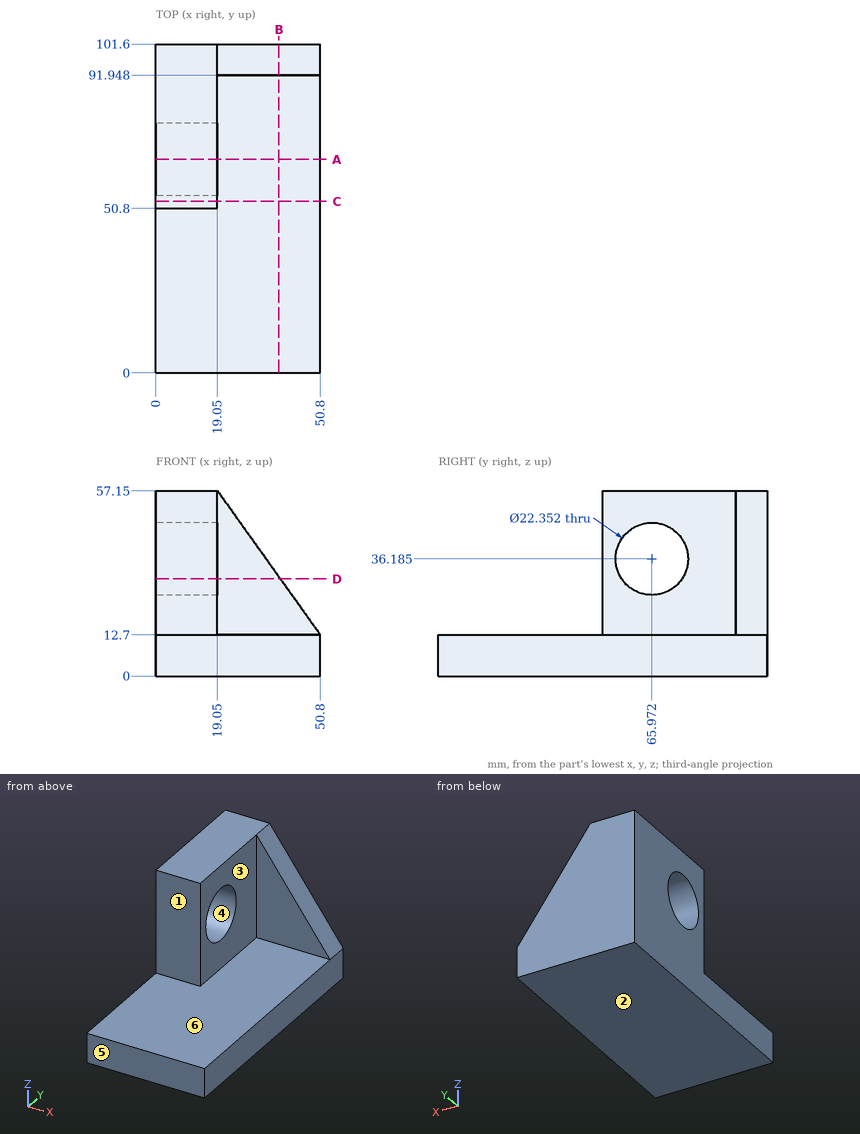
Verification items for this drawing (mm, ordinates from the low corner). A direction names the side the tool comes from. Give positions to 0.01 mm unless a question says otherwise; leave off trailing zeros. Loops run counter-clockwise (first coordinate to the right, second up) from the corner with the lowest first, then second, coordinate; pieces in that order, holes last. Notation, with made-up numbers: M 31.25,-33 L 49.25,-33 A27 cw 49.25,-16 Z; hole C 62.25,51.25 d8. An arc over 180 degrees is marked long. Answer as a JSON object with one key per item and string values. Group by question number.
Q1. Release check for a two-part mould opening along Y. For the marked faces 4, 5 and 6 record: released by +Y, released by -Y, zero draft, split by the parting line, or undercut.
Q2. Cross-section at B-B on x = 38. Record the cut outline in (y, z), then the cut area to 3 significant figures.
Q3. Access from +Z, -Z, +X, -X, +Y, -Y to the whole of each face (thin tool, end or side, straight path). Record for the marked faces 1, 2 and 3.
Q4. Cross-section at A-A on y = 66. Record the cut outline in (x, z).
Q5. Cross-section at C-C on y = 53. Record the cut outline in (x, z), then the cut area to 3 significant figures.
Q6. Go/stop test with flat-tipped pins: P1, Ø3, axis at x = 20.5, z = 42.5, coming from the -Y side; P2, Ø1.5, axis at y = 73.5, z = 16, coming from the +X side; P3, Ø1, axis at x = 24.5, y = 38.5, coming from the +Z side. Record where each tip stops, or that it passes through.
Q7. Cross-section at D-D on z = 30. Record the cut outline in (x, y).
Q8. Material ranges on line 1 along Y through (x, z) = (28, 37); line 2 along X through (y, z) = (83.5, 32.5); line 3 along Z through (x, y) = (14, 44), recorded low to high. Write a range as [from, to].
Evaluation:
{
 "1": {"face 4": "undercut", "face 5": "released by -Y", "face 6": "zero draft"},
 "2": {"outline": "M 0,0 L 101.6,0 L 101.6,30.62 L 91.95,30.62 L 91.95,12.7 L 0,12.7 Z", "area": "1,460 mm2"},
 "3": {"face 1": "+Z, +X, -X, -Y", "face 2": "-Z, +X, -X, +Y, -Y", "face 3": "+Z, +X, -Y"},
 "4": {"outline": "M 0,0 L 50.8,0 L 50.8,12.7 L 19.05,12.7 L 19.05,25.01 L 0,25.01 Z; M 0,47.36 L 19.05,47.36 L 19.05,57.15 L 0,57.15 Z"},
 "5": {"outline": "M 0,0 L 50.8,0 L 50.8,12.7 L 19.05,12.7 L 19.05,57.15 L 0,57.15 Z", "area": "1,490 mm2"},
 "6": {"P1": "stops at y = 50.8", "P2": "stops at x = 19.05", "P3": "stops at z = 12.7"},
 "7": {"outline": "M 0,50.8 L 19.05,50.8 L 19.05,56.66 L 0,56.66 Z; M 0,75.28 L 19.05,75.28 L 19.05,91.95 L 38.44,91.95 L 38.44,101.6 L 0,101.6 Z"},
 "8": {"line 1": "y = [91.95, 101.6]", "line 2": "x = [0, 19.05]", "line 3": "z = [0, 12.7]"}
}
